The figure shows three views and two pictorial views of one solid part (mm, origin at its lowest corner). Answer the questions. A direction names the side the tool comes from. Round coordinates to 2 decimals unless told otherwise and drop trailing zeros. Order: outer loops, then holes, each group sorted by start corner. A loop starts at its lowest first (then second) coordinate and runs counter-clockwise, first axis right, second up. Notation, with made-up numbers: (-0.75, -30.5) - (39.25, -30.5) arc R19 ccw to (39.25, 0.5) - close; hole circle Ø6 at (-20.75, 58.25). An arc over 180 degrees is marked (long way). Answer in a Markdown table with one row per item.
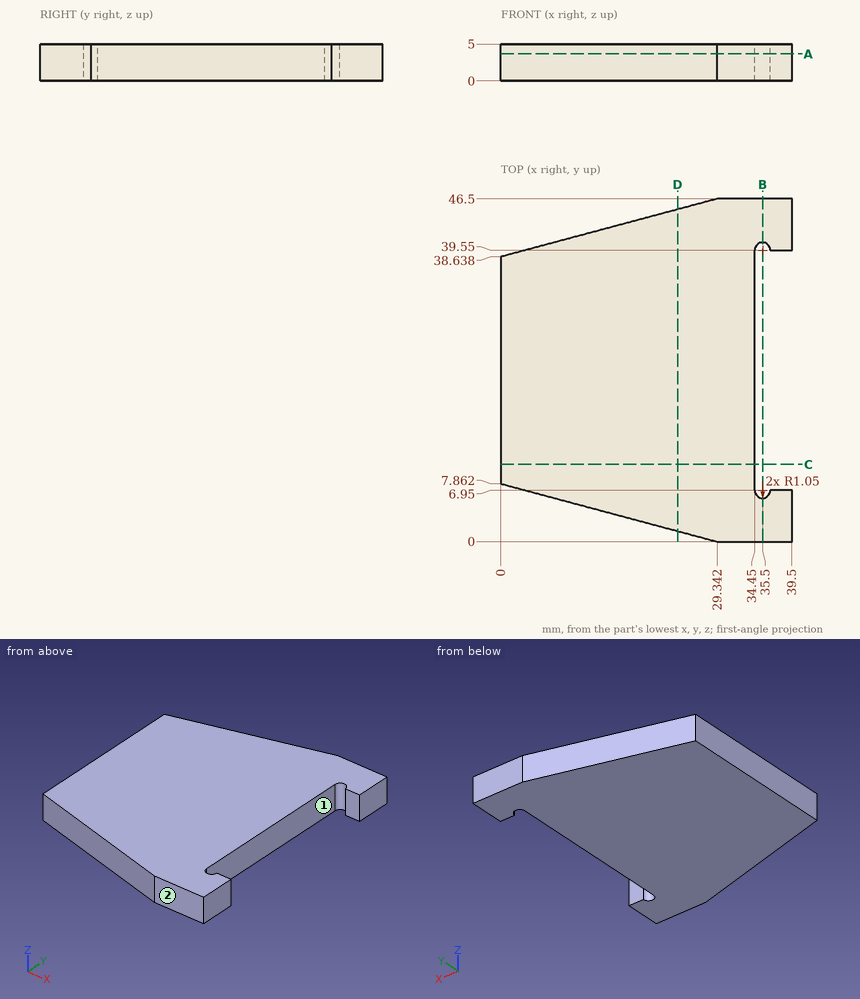
1) Find section A-A, the plane z = 3.65. Give the vertices of the cut face in (x, y), then the cut area to 3 significant figures.
Filled in:
| item | result |
|---|---|
| outline | (0, 7.86) - (29.34, 0) - (39.5, 0) - (39.5, 6.95) - (36.55, 6.95) arc R1.05 cw to (34.45, 6.95) - (34.45, 39.55) arc R1.05 cw to (36.55, 39.55) - (39.5, 39.55) - (39.5, 46.5) - (29.34, 46.5) - (0, 38.64) - close |
| area | 1,440 mm^2 |
2) Each of these flat-tipped pins is pushed along its axis until it touches: pin 1 (1 mm diameter, centred on x = 20, z = 1.5, fed in from -Y); pin 2 (1 mm diameter, centred on x = 25, z = 2, fed in from +Y); pin 3 (12 mm diameter, centred on x = 10, y = 27, fed in from -Z); pin 4 (1 mm diameter, centred on x = 22.5, z = 3.5, fed in from -Y). Where does it stop, or does it pass through?
Filled in:
| item | result |
|---|---|
| pin 1 | stops at y = 2.37 |
| pin 2 | stops at y = 45.47 |
| pin 3 | stops at z = 0 |
| pin 4 | stops at y = 1.7 |
3) Which of the six approach directions +Z, -Z, +X, -X, +Y, -Y give full straight-line access (tool end or side, diameter ignored) to the marked faces 1 and 2?
Filled in:
| item | result |
|---|---|
| face 1 | +Z, -Z, +X |
| face 2 | +Z, -Z, +X, -X, -Y |
4) Find section B-B, the plane x = 35.5. Give the vertices of the cut face in (y, z), then the cut area to 3 significant figures.
Filled in:
| item | result |
|---|---|
| outline | (0, 0) - (5.9, 0) - (5.9, 5) - (0, 5) - close; (40.6, 0) - (46.5, 0) - (46.5, 5) - (40.6, 5) - close |
| area | 59.0 mm^2 |
5) Find section D-D, the plane x = 24. Give the vertices of the cut face in (y, z).
Filled in:
| item | result |
|---|---|
| outline | (1.43, 0) - (45.07, 0) - (45.07, 5) - (1.43, 5) - close |
6) Find section C-C, the plane y = 10.5. Give the vertices of the cut face in (x, z).
Filled in:
| item | result |
|---|---|
| outline | (0, 0) - (34.45, 0) - (34.45, 5) - (0, 5) - close |
7) Find the intervals of material crossed by probe 1 along X at (y, z) = (35, 1.45); probe 2 along Y at (x, z) = (26.5, 1.3); probe 3 along Y at (x, z) = (9.5, 1.2), in increasing order. Write a range as from..to.
Filled in:
| item | result |
|---|---|
| probe 1 | x = 0..34.45 |
| probe 2 | y = 0.76..45.74 |
| probe 3 | y = 5.32..41.18 |
